The model under review builds one solid part; all positions refer to its coordinate system, in mm. A direction names the side the tool comes from. Coordinates: 2 decimals unless noted, no trailing zeros. Order: outer loops, then holes, each group sorted by start corner. A loop starts at its lowest first (then second) coordinate and runs counter-clockwise, first axis right, second up. Notation, with made-up numbers: (-37.75, 71.5) -> (-25.75, 71.5) arc R19 cw to (-25.75, 76.5) -> close; hole circle Ø4 at (59, 38.25). An arc over 180 degrees is marked (long way). Answer as CSV lines item,"result". Start each with the question number.
from build123d import *

# Parameters (mm, degrees)
PROFILE_DEPTH                               = 340.5
SKETCH2_W                                   = 8.5
SKETCH2_H                                   = 8.5
FEET_DEPTH                                  = 7
POCKETS_DEPTH                               = 355.98239393
RAIL_EDGE_R1_R                              = 1
M2_TAP_HOLES_SKETCH_R                       = 0.8
M2_TAP_HOLES_1_6_DRILL_DEPTH                = 355.98239393
FOOT_TAPS_SKETCH_Z0_END_R                   = 0.8
M2_FOOT_TAPS_1_6_DRILL_5_DEEP_Z0_END_DEPTH  = 5
M2_START                                    = -5
FOOT_TAPS_SKETCH_Z340_END_R                 = 0.8
M2_FOOT_TAPS_1_6_DRILL_5_DEEP_Z340_EN_DEPTH = 5
BRACES_DEPTH                                = 1.5
BRACES_2_DEPTH                              = 1.5
BRACES_OUTER_DEPTH                          = 1.5
BRACES_OUTER_2_DEPTH                        = 1.5
PANEL_PADS_SKETCH_W                         = 8
PANEL_PADS_SKETCH_H                         = 83
PANEL_PADS_DEPTH                            = 1.5


with BuildPart() as part:
    # Sketch1 → Profile (new body)
    with BuildSketch(Plane.XY):
        Polygon((0, 0), (0, 100), (8.5, 100), (8.5, 98.5), (1.5, 98.5), (1.5, 1.5), (8.5, 1.5), (8.5, 0), align=None)
    extrude(amount=PROFILE_DEPTH)

    # Sketch2 → Feet (add)
    with BuildSketch(Plane.XY):
        with Locations((4.25, 4.25)):
            Rectangle(SKETCH2_W, SKETCH2_H)
        with Locations((4.25, 95.75)):
            Rectangle(SKETCH2_W, SKETCH2_H)
    feet = extrude(amount=FEET_DEPTH)

    # Sketch5 → Pockets (cut, through all)
    with BuildSketch(Plane(origin=(0, 0, 0), x_dir=(0, 0, -1), z_dir=(1, 0, 0))):
        with BuildLine():
            Line((-15, 91.5), (-106.5, 91.5))
            ThreePointArc((-106.5, 91.5), (-108.621320344, 90.621320344), (-109.5, 88.5))
            Line((-109.5, 88.5), (-109.5, 11.5))
            ThreePointArc((-109.5, 11.5), (-108.621320344, 9.378679656), (-106.5, 8.5))
            Line((-106.5, 8.5), (-15, 8.5))
            ThreePointArc((-15, 8.5), (-12.878679656, 9.378679656), (-12, 11.5))
            Line((-12, 11.5), (-12, 88.5))
            ThreePointArc((-12, 88.5), (-12.878679656, 90.621320344), (-15, 91.5))
        make_face()
        with BuildLine():
            Line((-120.5, 91.5), (-220, 91.5))
            ThreePointArc((-220, 91.5), (-222.121320344, 90.621320344), (-223, 88.5))
            Line((-223, 88.5), (-223, 11.5))
            ThreePointArc((-223, 11.5), (-222.121320344, 9.378679656), (-220, 8.5))
            Line((-220, 8.5), (-120.5, 8.5))
            ThreePointArc((-120.5, 8.5), (-118.378679656, 9.378679656), (-117.5, 11.5))
            Line((-117.5, 11.5), (-117.5, 88.5))
            ThreePointArc((-117.5, 88.5), (-118.378679656, 90.621320344), (-120.5, 91.5))
        make_face()
        with BuildLine():
            Line((-234, 91.5), (-325.5, 91.5))
            ThreePointArc((-325.5, 91.5), (-327.621320344, 90.621320344), (-328.5, 88.5))
            Line((-328.5, 88.5), (-328.5, 11.5))
            ThreePointArc((-328.5, 11.5), (-327.621320344, 9.378679656), (-325.5, 8.5))
            Line((-325.5, 8.5), (-234, 8.5))
            ThreePointArc((-234, 8.5), (-231.878679656, 9.378679656), (-231, 11.5))
            Line((-231, 11.5), (-231, 88.5))
            ThreePointArc((-231, 88.5), (-231.878679656, 90.621320344), (-234, 91.5))
        make_face()
    extrude(amount=POCKETS_DEPTH, mode=Mode.SUBTRACT)

    # Rail Edge R1
    rail_edge_r1_edges = [part.edges().sort_by_distance(p)[0] for p in [
        (0, 0, 170.25),
        (0, 100, 170.25),
    ]]
    fillet(rail_edge_r1_edges, radius=RAIL_EDGE_R1_R)

    # Feet Mirror: Feet across plane
    add(feet.mirror(Plane.XY.offset(170.25)))

    # M2 tap holes sketch → M2 Tap Holes (1.6 drill) (cut, through all)
    with BuildSketch(Plane.XZ):
        with Locations((5, 20)):
            Circle(M2_TAP_HOLES_SKETCH_R)
        with Locations((5, 95.125)):
            Circle(M2_TAP_HOLES_SKETCH_R)
        with Locations((5, 170.25)):
            Circle(M2_TAP_HOLES_SKETCH_R)
        with Locations((5, 245.375)):
            Circle(M2_TAP_HOLES_SKETCH_R)
        with Locations((5, 320.5)):
            Circle(M2_TAP_HOLES_SKETCH_R)
    extrude(amount=-M2_TAP_HOLES_1_6_DRILL_DEPTH, mode=Mode.SUBTRACT)

    # Foot taps sketch z0 end → M2 Foot Taps (1.6 drill, 5 deep) z0 end (cut)
    with BuildSketch(Plane.XY.offset(7)):
        with Locations((4.5, 5.5)):
            Circle(FOOT_TAPS_SKETCH_Z0_END_R)
        with Locations((4.5, 94.5)):
            Circle(FOOT_TAPS_SKETCH_Z0_END_R)
    extrude(amount=-M2_FOOT_TAPS_1_6_DRILL_5_DEEP_Z0_END_DEPTH, mode=Mode.SUBTRACT)

    # Foot taps sketch z340 end → M2 Foot Taps (1.6 drill, 5 deep) z340 end (cut)
    with BuildSketch(Plane(origin=(0, 0, 333.5), x_dir=(-1, 0, 0), z_dir=(0, 0, -1)).offset(M2_START)):
        with Locations(Location((-4.5, 5.5, 0), (0, 0, 180))):
            Circle(FOOT_TAPS_SKETCH_Z340_END_R)
        with Locations(Location((-4.5, 94.5, 0), (0, 0, 180))):
            Circle(FOOT_TAPS_SKETCH_Z340_END_R)
    extrude(amount=M2_FOOT_TAPS_1_6_DRILL_5_DEEP_Z340_EN_DEPTH, mode=Mode.SUBTRACT)

    # Braces _ sketch → Braces (add)
    with BuildSketch(Plane.ZY):
        Polygon((13.944644974, 6.215627892), (111.444644974, 89.215627892), (107.555355026, 93.784372108), (10.055355026, 10.784372108), align=None)
        Polygon((119.354944806, 6.14220871), (224.854944806, 89.14220871), (221.145055194, 93.85779129), (115.645055194, 10.85779129), align=None)
        Polygon((232.944644974, 6.215627892), (330.444644974, 89.215627892), (326.555355026, 93.784372108), (229.055355026, 10.784372108), align=None)
    extrude(amount=-BRACES_DEPTH)

    # Braces _ sketch 2 → Braces 2 (add)
    with BuildSketch(Plane.ZY):
        Polygon((10.055355026, 89.215627892), (107.555355026, 6.215627892), (111.444644974, 10.784372108), (13.944644974, 93.784372108), align=None)
        Polygon((115.645055194, 89.14220871), (221.145055194, 6.14220871), (224.854944806, 10.85779129), (119.354944806, 93.85779129), align=None)
        Polygon((229.055355026, 89.215627892), (326.555355026, 6.215627892), (330.444644974, 10.784372108), (232.944644974, 93.784372108), align=None)
    extrude(amount=-BRACES_2_DEPTH)

    # Braces _ outer sketch → Braces _ outer (add)
    with BuildSketch(Plane.ZY):
        Polygon((13.944644974, 6.215627892), (111.444644974, 89.215627892), (107.555355026, 93.784372108), (10.055355026, 10.784372108), align=None)
        Polygon((119.354944806, 6.14220871), (224.854944806, 89.14220871), (221.145055194, 93.85779129), (115.645055194, 10.85779129), align=None)
        Polygon((232.944644974, 6.215627892), (330.444644974, 89.215627892), (326.555355026, 93.784372108), (229.055355026, 10.784372108), align=None)
    extrude(amount=BRACES_OUTER_DEPTH)

    # Braces _ outer sketch 2 → Braces _ outer 2 (add)
    with BuildSketch(Plane.ZY):
        Polygon((10.055355026, 89.215627892), (107.555355026, 6.215627892), (111.444644974, 10.784372108), (13.944644974, 93.784372108), align=None)
        Polygon((115.645055194, 89.14220871), (221.145055194, 6.14220871), (224.854944806, 10.85779129), (119.354944806, 93.85779129), align=None)
        Polygon((229.055355026, 89.215627892), (326.555355026, 6.215627892), (330.444644974, 10.784372108), (232.944644974, 93.784372108), align=None)
    extrude(amount=BRACES_OUTER_2_DEPTH)

    # Panel pads sketch → Panel pads (add)
    with BuildSketch(Plane.ZY):
        with Locations((8, 50)):
            Rectangle(PANEL_PADS_SKETCH_W, PANEL_PADS_SKETCH_H)
        with Locations((113.5, 50)):
            Rectangle(PANEL_PADS_SKETCH_W, PANEL_PADS_SKETCH_H)
        with Locations((227, 50)):
            Rectangle(PANEL_PADS_SKETCH_W, PANEL_PADS_SKETCH_H)
        with Locations((332.5, 50)):
            Rectangle(PANEL_PADS_SKETCH_W, PANEL_PADS_SKETCH_H)
    extrude(amount=PANEL_PADS_DEPTH)


solid = part.part
1) Wall thickness on L1, parallel to Y at x = 4.5, z = 4.4; L2, parallel to Z at x = 5, y = 0.85 (3 decimals); L3, parallel to Y at x = 3.5, z = 243.5: over which ranges is each line inside the solid? List them lowest first. Write a range as [from, to].
2) Insertion check: pin 1 Ø1.8 at (x, z) = (5, 245.375) entering from -Y; pin 2 Ø0.8 at (x, z) = (-0.5, 112.5) entering from +Y. Each pin has a flat end and moves straight along its axis. Give the tip position at first contact, or say it passes through.
3) Consider section B-B (y = 76). Count the separate pieces of the cut face and the enclosed holes in it, plus the area to 3 significant figures.
4) Mouldability with a two-part tool opening along Y and no side actions: class faces 1 (the face through (4, 0, 173)), 2 (the face through (1, 51, 0)), 3 (the face through (0.021, 26.417, 302.825)) as released by +Y, released by -Y, zero draft, split by the parting line, or undercut.
5) Consider section A-A (z = 311). Give the boundary of the cut face in (x, y), plus the area to 3 significant figures.
6) Tool access review of faces 4 (the face through (0.02, 69.11, 141.11)), 5 (the face through (5, 98.5, 168)), 6 (the face through (5, 91.5, 337)): name each direction out of +Z, -Z, +X, -X, +Y, -Y from which nothing blocks a thin tool from reaching the whole face with its end or side.
Result:
1,L1,"[0, 4.7], [6.3, 8.5], [91.5, 93.7], [95.3, 100]"
1,L2,"[0, 19.2], [20.8, 94.325], [95.925, 169.45], [171.05, 244.575], [246.175, 319.7], [321.3, 340.5]"
1,L3,"[0, 1.5], [98.5, 100]"
2,pin 1,"y = 0"
2,pin 2,"y = 91.5"
3,separate pieces,"10"
3,enclosed holes,"0"
3,area,"277 mm2"
4,face 1,"released by -Y"
4,face 2,"zero draft"
4,face 3,"undercut"
5,outline,"(-1.5, 19.46) -> (1.5, 19.46) -> (1.5, 27.34) -> (-1.5, 27.34) -> close; (-1.5, 72.66) -> (1.5, 72.66) -> (1.5, 80.54) -> (-1.5, 80.54) -> close; (0, 1) arc R1 ccw to (1, 0) -> (8.5, 0) -> (8.5, 1.5) -> (1.5, 1.5) -> (1.5, 8.5) -> (0, 8.5) -> close; (0, 91.5) -> (1.5, 91.5) -> (1.5, 98.5) -> (8.5, 98.5) -> (8.5, 100) -> (1, 100) arc R1 ccw to (0, 99) -> close"
5,area,"93.3 mm2"
6,face 4,"+X, -X"
6,face 5,"+X"
6,face 6,"+Z, -Z, +X"
